from build123d import *

# Parameters (mm, degrees)
SKETCH2_R           = 127
SKETCH2_R_2         = 6
SKETCH2_R_3         = 31.75
BOSS_EXTRUDE1_DEPTH = 6.35
SCALE1_SCALE        = 0.714781685
SCALE2_SCALE        = 0.5
BOSS_EXTRUDE2_START = -4.538863701
SKETCH3_R           = 11.347159253
SKETCH3_R_2         = 10.05
BOSS_EXTRUDE2_DEPTH = 4.538863701
SCALE3_SCALE        = 1.5
BOSS_EXTRUDE3_START = -6.808295552
SKETCH4_R           = 15.075
SKETCH4_R_2         = 10.05
BOSS_EXTRUDE3_DEPTH = 6.808295552


with BuildPart() as part:
    # Sketch2 → Boss-Extrude1 (new, symmetric)
    with BuildSketch(Plane(origin=(0, 0, 0), x_dir=(0, 0, -1), z_dir=(1, 0, 0))):
        Circle(SKETCH2_R)
        with Locations((-82.709756188, 47.7525)):
            Circle(SKETCH2_R_2, mode=Mode.SUBTRACT)
        with Locations((-35.943005468, 88.483362181)):
            Circle(SKETCH2_R_2, mode=Mode.SUBTRACT)
        with Locations((-82.709756188, -47.7525)):
            Circle(SKETCH2_R_2, mode=Mode.SUBTRACT)
        with Locations((-94.600342195, 13.114125267)):
            Circle(SKETCH2_R_2, mode=Mode.SUBTRACT)
        with Locations((0, -95.505)):
            Circle(SKETCH2_R_2, mode=Mode.SUBTRACT)
        with Locations((-58.657336727, -75.369236914)):
            Circle(SKETCH2_R_2, mode=Mode.SUBTRACT)
        with Locations((82.709756188, -47.7525)):
            Circle(SKETCH2_R_2, mode=Mode.SUBTRACT)
        with Locations((35.943005468, -88.483362181)):
            Circle(SKETCH2_R_2, mode=Mode.SUBTRACT)
        with Locations((82.709756188, 47.7525)):
            Circle(SKETCH2_R_2, mode=Mode.SUBTRACT)
        with Locations((94.600342195, -13.114125267)):
            Circle(SKETCH2_R_2, mode=Mode.SUBTRACT)
        with Locations((58.657336727, 75.369236914)):
            Circle(SKETCH2_R_2, mode=Mode.SUBTRACT)
        with Locations((0, 95.505)):
            Circle(SKETCH2_R_2, mode=Mode.SUBTRACT)
        Circle(SKETCH2_R_3, mode=Mode.SUBTRACT)
    extrude(amount=BOSS_EXTRUDE1_DEPTH, both=True)


with BuildPart() as part_1:
    # Scale1: scaled about (0, 0, 0)
    add(part.part.scale(SCALE1_SCALE))


with BuildPart() as part_2:
    # Scale2: scaled about (0, 0, 0)
    add(part_1.part.scale(SCALE2_SCALE))

    # Sketch3 → Boss-Extrude2 (add)
    with BuildSketch(Plane(origin=(2.269431851, 0, 0), x_dir=(0, 0, -1), z_dir=(1, 0, 0)).offset(BOSS_EXTRUDE2_START)):
        Circle(SKETCH3_R)
        Circle(SKETCH3_R_2, mode=Mode.SUBTRACT)
    extrude(amount=BOSS_EXTRUDE2_DEPTH)


with BuildPart() as part_3:
    # Scale3: scaled about (0, 0, 0)
    add(part_2.part.scale(SCALE3_SCALE))

    # Sketch4 → Boss-Extrude3 (add)
    with BuildSketch(Plane(origin=(3.404147776, 0, 0), x_dir=(0, 0, -1), z_dir=(1, 0, 0)).offset(BOSS_EXTRUDE3_START)):
        Circle(SKETCH4_R)
        Circle(SKETCH4_R_2, mode=Mode.SUBTRACT)
    extrude(amount=BOSS_EXTRUDE3_DEPTH)


solid = part_3.part
Design review of the part built by this model. Coordinates are the model's own, in mm. Coordinates: 2 decimals unless noted, no trailing zeros. Loops run counter-clockwise (first coordinate to the right, second up) from the corner with the lowest first, then second, coordinate; pieces in that order, holes last. Notation, with made-up numbers: M -24,33.5 L 19,33.5 A35 cw 19,71.5 Z; hole C -34.5,-0.5 d9. An arc over 180 degrees is marked long. Answer as CSV lines item,"result".
Item 1: For probe 1 along Y at (x, z) = (-0.75, 0); probe 2 along Z at (x, y) = (3, 0.5); probe 3 along Y at (x, z) = (2, -46), list the stretches that pass through material, from the lowest coordinate up.
Answer list:
probe 1,"-68.08 to -54.42, -47.98 to -10.05, 10.05 to 47.98, 54.42 to 68.08"
probe 2,"-68.08 to -10.04, 10.04 to 68.08"
probe 3,"-50.19 to -28.35, -22.84 to 22.84, 28.35 to 50.19"
Item 2: The part is to be moulded in two halves that separate along Y. For faces 1 (the face through (-0.05, 23.64, 46.89)), 2 (the face through (-0.05, -22.41, 44.76)), 3 (the face through (0.048, -66.464, 14.759)), 4 (the face through (3.404, -14, 1)), say which applies: pulls with the +Y half, pulls with the -Y half, needs draft (parallel to the pull), parting line crosses it, or undercut.
Answer list:
face 1,"undercut"
face 2,"undercut"
face 3,"parting line crosses it"
face 4,"needs draft"
Item 3: Add section D-D on x = -2. Count the separate pieces of the cut face and the enclosed holes in it, plus the area to 3 significant figures.
Answer list:
separate pieces,"1"
enclosed holes,"13"
area,"13,900 mm²"
Item 4: Add section A-A on z = 0. State the section outline as (x, y) points, plus the area to 3 significant figures.
Answer list:
outline,"M -3.4,-68.08 L 3.4,-68.08 L 3.4,-54.42 L -3.4,-54.42 Z; M -3.4,-47.98 L 3.4,-47.98 L 3.4,-10.05 L -3.4,-10.05 Z; M -3.4,10.05 L 3.4,10.05 L 3.4,47.98 L -3.4,47.98 Z; M -3.4,54.42 L 3.4,54.42 L 3.4,68.08 L -3.4,68.08 Z"
area,"703 mm²"
Item 5: Add section B-B on y = 0. State the section outline as (x, z) points.
Answer list:
outline,"M -3.4,-68.08 L 3.4,-68.08 L 3.4,-10.05 L -3.4,-10.05 Z; M -3.4,10.05 L 3.4,10.05 L 3.4,68.08 L -3.4,68.08 Z"
Item 6: Add section C-C on z = 19. State the section outline as (x, y) points.
Answer list:
outline,"M -3.4,-65.38 L 3.4,-65.38 L 3.4,44.23 L -3.4,44.23 Z; M -3.4,50.64 L 3.4,50.64 L 3.4,65.38 L -3.4,65.38 Z"
Item 7: For P1, Ø4, axis at y = 51.2, z = 0, coming from the +X side; P2, Ø3, axis at x = 1.5, y = -23.5, coming from the -Z side; P3, Ø3, axis at x = -0.5, z = -54, coming from the -Y side, all flat-tipped, find the tip position at first contact; note any pin that passes through.
Answer list:
P1,"through"
P2,"z = -64.43"
P3,"y = -43.35"
